CAD build for the part. Positions are in the model's coordinates, mm. A direction names the side the tool comes from. Coordinates: 2 decimals unless noted, no trailing zeros. Order: outer loops, then holes, each group sorted by start corner. A loop starts at its lowest first (then second) coordinate and runs counter-clockwise, first axis right, second up. Notation, with made-up numbers: M -4.75,24 L 27.25,24 A38 cw 27.25,62 Z; hole C 83.5,31 d7. An arc over 180 degrees is marked long. One line per item, written item: value.
from build123d import *

# Parameters (mm, degrees)
SKETCH_1_R      = 11.5
EXTRUDE_1_DEPTH = 10
SKETCH_2_R      = 8.5
EXTRUDE_2_DEPTH = 10
SKETCH_3_R      = 4
EXTRUDE_3_DEPTH = 2
SKETCH_4_R      = 5
EXTRUDE_4_DEPTH = 13
CHAMFER_1_SIZE  = 2
CHAMFER_2_SIZE  = 1


with BuildPart() as part:
    # 草图1 → 拉伸1 (new body)
    with BuildSketch(Plane.XY):
        Circle(SKETCH_1_R)
    extrude(amount=EXTRUDE_1_DEPTH)

    # 草图2 → 拉伸2 (add)
    with BuildSketch(Plane.XY.offset(10)):
        Circle(SKETCH_2_R)
    extrude(amount=EXTRUDE_2_DEPTH)

    # 草图3 → 拉伸3 (add)
    with BuildSketch(Plane.XY.offset(20)):
        Circle(SKETCH_3_R)
    extrude(amount=EXTRUDE_3_DEPTH)

    # 草图4 → 拉伸4 (add)
    with BuildSketch(Plane.XY.offset(22)):
        with Locations(Location((0, 0, 0), (0, 0, 180))):
            Circle(SKETCH_4_R)
    extrude(amount=EXTRUDE_4_DEPTH)

    # 草图6 → 切除-旋转1 (revolve, cut)
    with BuildSketch(Plane(origin=(0, 0, 0), x_dir=(1, 0, 0), z_dir=(0, 1, 0))):
        Polygon((0, -35), (2, -35), (2, -15), (0, -13.845299462), align=None)
    revolve(axis=Axis((0, 0, 2.170078688), (0, 0, 1)), mode=Mode.SUBTRACT)

    # 草图7 → 切除-旋转2 (revolve, cut)
    with BuildSketch(Plane(origin=(0, 0, 0), x_dir=(1, 0, 0), z_dir=(0, 1, 0))):
        Polygon((-8.5, -15), (-8.5, -17), (3.5, -17), (4.654700538, -15), align=None)
    revolve(axis=Axis((-16.340863748, 0, 15), (1, 0, 0)), mode=Mode.SUBTRACT)

    # 倒角1
    chamfer_1_edges = [part.edges().sort_by_distance(p)[0] for p in [
        (-11.5, 0, 0),
        (-11.5, 0, 10),
    ]]
    chamfer(chamfer_1_edges, length=CHAMFER_1_SIZE)

    # 倒角2
    chamfer_2_edges = [part.edges().sort_by_distance(p)[0] for p in [
        (5, 0, 35),
    ]]
    chamfer(chamfer_2_edges, length=CHAMFER_2_SIZE)


solid = part.part
Q1. Mould opens along Y. For faces 1 (the face through (4.47, 0.194, 14.747)), 2 (the face through (-0.867, -3.905, 20.986)), 3 (the face through (0, 0, 0)) say: released by +Y, released by -Y, zero draft, split by the parting line, or undercut.
Recorded:
face 1: undercut
face 2: split by the parting line
face 3: zero draft
Q2. Slice it at C-C (z = 10.5). List the corners of the cut face in (x, y), plus the area to 3 significant figures.
Recorded:
outline: C 0,0 d17
area: 227 mm^2
Q3. Slice it at A-A (x = 0). List the corners of the cut face in (y, z), plus the area to 3 significant figures.
Recorded:
outline: M -11.5,2 L -9.5,0 L 9.5,0 L 11.5,2 L 11.5,8 L 9.5,10 L 8.5,10 L 8.5,20 L 4,20 L 4,22 L 5,22 L 5,34 L 4,35 L 2,35 L 2,15 A2 cw -2,15 L -2,35 L -4,35 L -5,34 L -5,22 L -4,22 L -4,20 L -8.5,20 L -8.5,10 L -9.5,10 L -11.5,8 Z
area: 451 mm^2
Q4. Drill centre lines: line 1 along Z through (x, y) = (3, 9); line 2 along Y through (x, z) = (0, 30.75); line 3 along Y through (x, z) = (0, 21.5). Where is each one in solid material? Low to high.
Recorded:
line 1: z = 0 to 10
line 2: y = -5 to -2, 2 to 5
line 3: y = -4 to -2, 2 to 4
Q5. Which spindle directions (+Z, -Z, +X, -X, +Y, -Y) get a long thin tool onto all of the face, cutting with end or side? Do faces 4 (the face through (-1.5, 11.4, 5)), 5 (the face through (4, -2, 20)), 6 (the face through (-2, 0, 13)), 7 (the face through (5, 0, 28)), 8 (the face through (2, 1, 35)). Say none if no direction does.
Recorded:
face 4: +Z, -Z
face 5: none
face 6: -X
face 7: +Z
face 8: +Z, +X, -X, +Y, -Y
Q6. Pin check, flat tips, straight feed: pin 1 Ø3.5 at (x, y) = (0, 0) entering from +Z; pin 2 Ø5 at (x, z) = (0.5, 26) entering from +Y; pin 3 Ø5 at (y, z) = (0, 15) entering from -X; pin 4 Ø6 at (x, z) = (9, 28.5) entering from -Y. Stop position of each tip, or through.
Recorded:
pin 1: stops at z = 14.03
pin 2: stops at y = 5
pin 3: stops at x = -8.5
pin 4: passes through
Q7. Slice it at B-B (z = 28). List the corners of the cut face in (x, y), plus the area to 3 significant figures.
Recorded:
outline: C 0,0 d10; hole C 0,0 d4
area: 66.0 mm^2
